The listing builds one solid part. Answer for the finished solid, in the listing's coordinates (mm). Give positions to 0.01 mm unless a question says otherwise; leave off trailing zeros. Order: outer loops, then holes, each group sorted by start corner. A loop starts at its lowest first (then second) coordinate and runs counter-clockwise, first axis right, second up. Notation, with made-up numbers: (83, 50) - (95, 50) arc R21 ccw to (95, 80) - close; hole circle Ø3 at (-10, 50). An arc over 180 degrees is marked (long way). Use a Markdown table: item, result. Add a question column.
1) Find section A-A, the plane x = 3. Determine the outline of the cut face in (y, z).
2) Find section B-B, the plane x = 51.5. Determine the outline of the cut face in (y, z).
3) Find section D-D, the plane x = 23. Determine the outline of the cut face in (y, z), plus the area to 3 significant figures.
4) Straight lines are drawn through the part: line 1 (Y direction, x = -13.5, z = 1.2); line 2 (X direction, y = 5.5, z = 0.4); line 3 (Y direction, x = -0.5, z = 0.7). For each, find the intervals that lie inside material, in ascending order.
5) Find section C-C, the plane y = 24. Determine the outline of the cut face in (x, z).
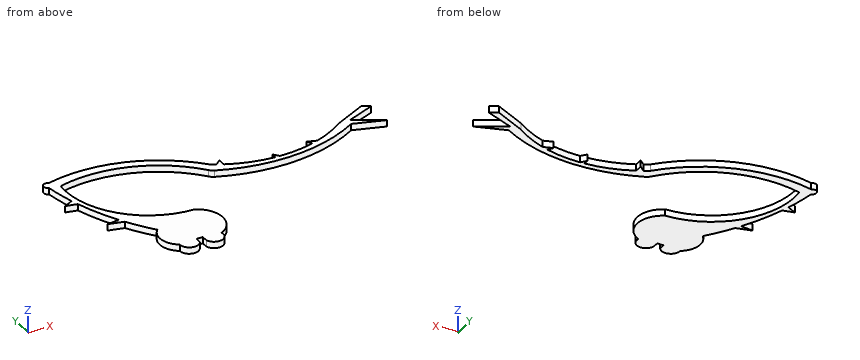
from build123d import *

# Parameters (mm, degrees)
BOSS_EXTRUDE1_DEPTH = 1.524


with BuildPart() as part:
    # Sketch1 → Boss-Extrude1 (new body)
    with BuildSketch(Plane.XY):
        with BuildLine():
            ThreePointArc((-16.197076151, 32.337475868), (-17.011067411, 35.784074673), (-17.596756232, 39.276723195))
            ThreePointArc((-17.596756232, 39.276723195), (-18.186455817, 40.773995588), (-16.610546214, 41.09969352))
            ThreePointArc((-16.610546214, 41.09969352), (1.114796248, 40.752315398), (16.047100727, 31.195395396))
            ThreePointArc((16.047100727, 31.195395396), (16.65383311, 30.831484379), (17.269539256, 30.482971317))
            Line((17.269539256, 30.482971317), (18.609894912, 31.696837019))
            Line((18.609894912, 31.696837019), (18.609894912, 29.792589361))
            ThreePointArc((18.609894912, 29.792589361), (23.848153012, 27.88417162), (29.360160247, 27.048000318))
            Line((29.360160247, 27.048000318), (29.360160247, 28.312908217))
            Line((29.360160247, 28.312908217), (30.371964085, 27.014480945))
            ThreePointArc((30.371964085, 27.014480945), (34.609173407, 27.271356348), (38.759272861, 28.163882163))
            Line((38.759272861, 28.163882163), (38.063395752, 29.375894853))
            Line((38.063395752, 29.375894853), (40.24389972, 28.648108402))
            ThreePointArc((40.24389972, 28.648108402), (44.068672668, 30.34536008), (47.598834428, 32.592026348))
            Line((47.598834428, 32.592026348), (55.083699621, 36.417717956))
            Line((55.083699621, 36.417717956), (56.910260303, 35.388944708))
            Line((56.910260303, 35.388944708), (50.185076604, 32.592026348))
            Line((50.185076604, 32.592026348), (56.910260303, 28.804203066))
            Line((56.910260303, 28.804203066), (49.712738856, 31.130827352))
            ThreePointArc((49.712738856, 31.130827352), (33.020763696, 25.765572392), (15.708965282, 28.542194647))
            ThreePointArc((15.708965282, 28.542194647), (15.163131597, 28.853301218), (14.710356917, 29.288866136))
            ThreePointArc((14.710356917, 29.288866136), (1.215411603, 38.505400506), (-15.123980563, 38.792312441))
            ThreePointArc((-15.123980563, 38.792312441), (-10.396030461, 23.399793439), (4.263099046, 16.736980561))
            ThreePointArc((4.263099046, 16.736980561), (7.676752936, 11.186831392), (4.263099046, 5.636682223))
            ThreePointArc((4.263099046, 5.636682223), (2.666546478, 2.970135745), (0, 4.566688313))
            Line((0, 4.566688313), (0, 6.017862143))
            Line((0, 6.017862143), (-1.524, 6.017862143))
            Line((-1.524, 6.017862143), (-1.524, 4.566688313))
            ThreePointArc((-1.524, 4.566688313), (-4.040524665, 3.505966865), (-5.665097739, 5.701140823))
            ThreePointArc((-5.665097739, 5.701140823), (-7.938147597, 9.268051635), (-6.680633826, 13.306401238))
            ThreePointArc((-6.680633826, 13.306401238), (-8.875864768, 16.330833019), (-10.856041848, 19.50023757))
            Line((-10.856041848, 19.50023757), (-14.485790124, 20.389849107))
            Line((-14.485790124, 20.389849107), (-11.572605425, 20.780961266))
            ThreePointArc((-11.572605425, 20.780961266), (-13.878489207, 25.592275915), (-15.696943684, 30.608157889))
            Line((-15.696943684, 30.608157889), (-18.384655546, 31.195395396))
            Line((-18.384655546, 31.195395396), (-16.197076151, 32.337475868))
        make_face()
    extrude(amount=BOSS_EXTRUDE1_DEPTH)


solid = part.part
The answers:
| question | item | result |
|---|---|---|
| 1 | outline | (3.08, 0) - (16.78, 0) - (16.78, 1.52) - (3.08, 1.52) - close; (37.87, 0) - (40.12, 0) - (40.12, 1.52) - (37.87, 1.52) - close |
| 2 | outline | (30.55, 0) - (31.85, 0) - (31.85, 1.52) - (30.55, 1.52) - close; (33.14, 0) - (34.59, 0) - (34.59, 1.52) - (33.14, 1.52) - close |
| 3 | outline | (26.34, 0) - (28.11, 0) - (28.11, 1.52) - (26.34, 1.52) - close |
| 3 | area | 2.70 mm2 |
| 4 | line 1 | 20.15 to 20.52, 24.71 to 28.19, 39.2 to 41.75 |
| 4 | line 2 | -5.66 to -1.52, 0 to 4.29 |
| 4 | line 3 | 6.02 to 17.34, 38.99 to 41.2 |
| 5 | outline | (-13.18, 0) - (-10.9, 0) - (-10.9, 1.52) - (-13.18, 1.52) - close |
